Here's how the part is built. I have some questions about the finished solid (model axes, mm). A direction names the side the tool comes from. Round coordinates to 2 decimals unless told otherwise and drop trailing zeros. Write each loop counter-clockwise with the first axis right and the second up, starting at its lowest first coordinate (ties: lowest second). Pieces come first, ordered by that corner, then holes. Notation, with made-up numbers: (21, 16.25) -> (51, 16.25) arc R16 cw to (51, 27.25) -> close; hole circle Ø1 at (45, 22). An arc over 180 degrees is marked (long way). Answer as CSV lines item,"result".
```python
from build123d import *

# Parameters (mm, degrees)
SKETCH1_R           = 7.5
BOSS_EXTRUDE1_DEPTH = 150
CUT_EXTRUDE1_START  = -9
SKETCH2_R           = 7.5
SKETCH2_R_2         = 6
CUT_EXTRUDE1_DEPTH  = 9
SKETCH3_R           = 3.5
CUT_EXTRUDE2_DEPTH  = 20


with BuildPart() as part:
    # Sketch1 → Boss-Extrude1 (new body)
    with BuildSketch(Plane.XY):
        Circle(SKETCH1_R)
    extrude(amount=BOSS_EXTRUDE1_DEPTH)

    # Sketch2 → Cut-Extrude1 (cut)
    with BuildSketch(Plane.XY.offset(150).offset(CUT_EXTRUDE1_START)):
        Circle(SKETCH2_R)
        Circle(SKETCH2_R_2, mode=Mode.SUBTRACT)
    extrude(amount=CUT_EXTRUDE1_DEPTH, mode=Mode.SUBTRACT)

    # Sketch3 → Cut-Extrude2 (cut)
    with BuildSketch(Plane.XY.offset(150)):
        Circle(SKETCH3_R)
    extrude(amount=-CUT_EXTRUDE2_DEPTH, mode=Mode.SUBTRACT)


solid = part.part
```
1. Suppose I cut it at C-C on z = 52. Please give me the cut outline in (x, y), and give its area (3 significant figures).
Numbers:
outline,"circle Ø15 at (0, 0)"
area,"177 mm^2"
2. If I drill on line 1 (Y direction, x = 0, z = 144.25); line 2 (Z direction, x = -1, y = 1.5); line 3 (Z direction, x = -6.5, y = -1.5), over which ranges is the centre line in solid material (lowest first)?
Numbers:
line 1,"y = -6 to -3.5, 3.5 to 6"
line 2,"z = 0 to 130"
line 3,"z = 0 to 141"
3. For pin 1 Ø3 at (x, z) = (-5, 66.5) entering from -Y; pin 2 Ø5 at (y, z) = (-3, 71.5) entering from -X; pin 3 Ø2 at (x, y) = (-1, -1) entering from +Z; pin 4 Ø8 at (x, z) = (-0.5, 134.5) entering from +Y, each with a flat end and sliding along its axis, tell me the tip position at first contact or that it passes through.
Numbers:
pin 1,"stops at y = -6.63"
pin 2,"stops at x = -7.48"
pin 3,"stops at z = 130"
pin 4,"stops at y = 7.5"
4. Suppose I cut it at A-A on x = 0. Please give me the cut outline in (y, z).
Numbers:
outline,"(-7.5, 0) -> (7.5, 0) -> (7.5, 141) -> (6, 141) -> (6, 150) -> (3.5, 150) -> (3.5, 130) -> (-3.5, 130) -> (-3.5, 150) -> (-6, 150) -> (-6, 141) -> (-7.5, 141) -> close"
5. On a 3-axis mill with a long thin cutter (end or side, diameter ignored), from which of +Z, -Z, +X, -X, +Y, -Y can I reach the whole of each face in a straight line? I mean faces 4 (the face through (3, -3, 150)), 5 (the face through (-6, 0, 145)). Say none if no direction works.
Numbers:
face 4,"+Z, +X, -X, +Y, -Y"
face 5,"+Z"
6. If we mould it in two halves opening along X, with no side actions, what happens to faces 1 (the face through (0, 0, 130)), 2 (the face through (2, 6, 141)), 3 (the face through (-7.493, 0.33, 69.513))? For each: released by +X, released by -X, zero draft, split by the parting line, or undercut.
Numbers:
face 1,"undercut"
face 2,"zero draft"
face 3,"split by the parting line"
